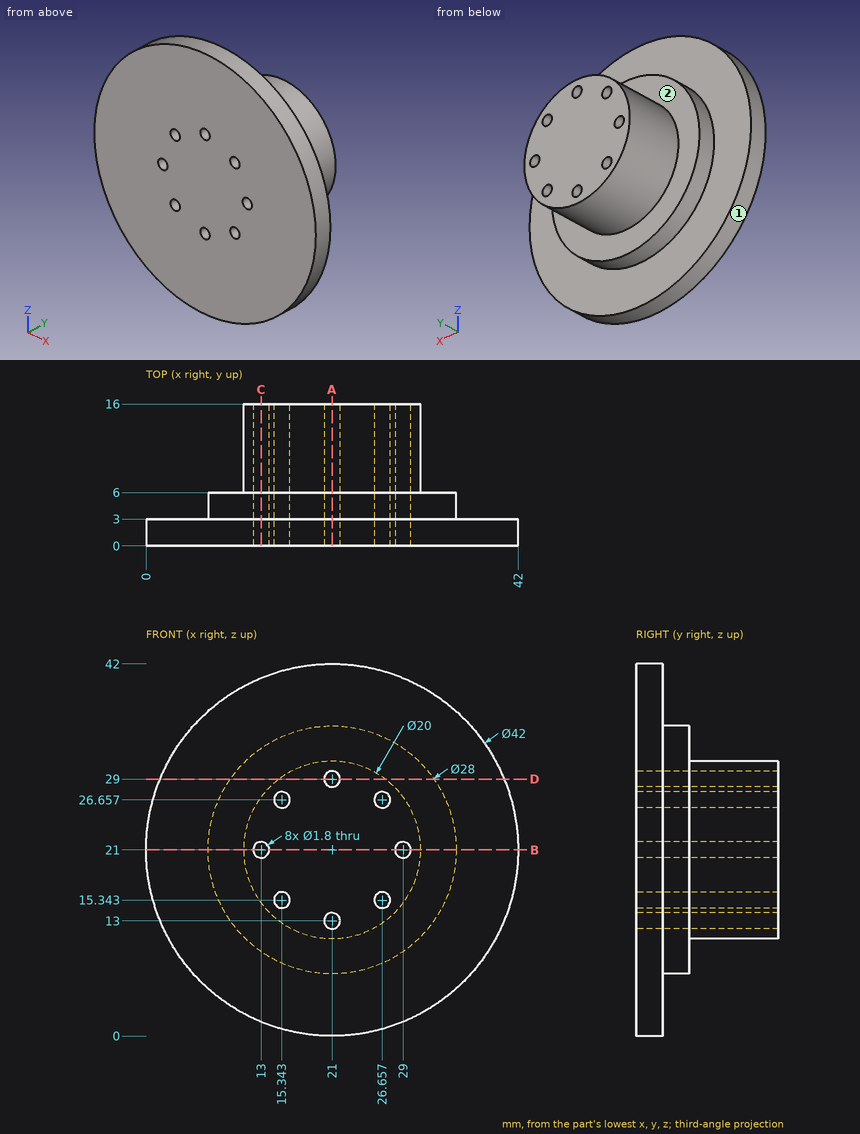
The drawing under review shows one solid part. Ordinate dimensions are in mm from its lowest x, y, z. A direction names the side the tool comes from. Coordinates: 2 decimals unless noted, no trailing zeros. Loops run counter-clockwise (first coordinate to the right, second up) from the corner with the lowest first, then second, coordinate; pieces in that order, holes last. Notation, with made-up numbers: (-24, 44.25) - (3, 44.25) arc R11 ccw to (3, 50.25) - close; hole circle Ø8 at (-39, 14.5). An arc over 180 degrees is marked (long way). Use CSV: the item, a comma, the result in double quotes. Start each with the question number.
1. Add section B-B on z = 21. Give the boundary of the cut face in (x, y).
2. Clearance check with flat-ended pins moving along their axes: pin 1 (2 mm diameter, centred on y = 12, z = 17.5, fed in from -X); pin 2 (4 mm diameter, centred on x = 25.5, z = 6.5, fed in from +Y); pin 3 (5 mm diameter, centred on y = 4, z = 14, fed in from -X). State where each tip first meets the part, or that it passes through.
3. Add section A-A on x = 21. Give the boundary of the cut face in (y, z).
4. Add section D-D on z = 29. Give the boundary of the cut face in (x, y).
5. To check wall thickness, follow probe 1 along Z at (x, y) = (21, 3.75); probe 2 along Y at (x, z) = (36.5, 32); probe 3 along X at (y, z) = (6.5, 16). State the ranges of each line that lie inside material, in increasing order.
6. Add section C-C on x = 13. Give the boundary of the cut face in (y, z), plus the area to 3 significant figures.
7. For the marked faces 1 and 2, list the 3-axis set-ups (+Z, -Z, +X, -X, +Y, -Y) from which the entire face can be reached by the end or side of a thin tool; tool diameter is ignored.
Resolved:
1,outline,"(0, 0) - (12.1, 0) - (12.1, 16) - (11, 16) - (11, 6) - (7, 6) - (7, 3) - (0, 3) - close; (13.9, 0) - (28.1, 0) - (28.1, 16) - (13.9, 16) - close; (29.9, 0) - (42, 0) - (42, 3) - (35, 3) - (35, 6) - (31, 6) - (31, 16) - (29.9, 16) - close"
2,pin 1,"x = 11.32"
2,pin 2,"y = 6"
2,pin 3,"x = 0.53"
3,outline,"(0, 0) - (3, 0) - (3, 7) - (6, 7) - (6, 11) - (16, 11) - (16, 12.1) - (0, 12.1) - close; (0, 13.9) - (16, 13.9) - (16, 28.1) - (0, 28.1) - close; (0, 29.9) - (16, 29.9) - (16, 31) - (6, 31) - (6, 35) - (3, 35) - (3, 42) - (0, 42) - close"
4,outline,"(1.58, 0) - (20.1, 0) - (20.1, 16) - (15, 16) - (15, 6) - (9.51, 6) - (9.51, 3) - (1.58, 3) - close; (21.9, 0) - (40.42, 0) - (40.42, 3) - (32.49, 3) - (32.49, 6) - (27, 6) - (27, 16) - (21.9, 16) - close"
5,probe 1,"7 to 12.1, 13.9 to 28.1, 29.9 to 35"
5,probe 2,"0 to 3"
5,probe 3,"12.34 to 14.73, 15.96 to 26.04, 27.27 to 29.66"
6,outline,"(0, 1.58) - (3, 1.58) - (3, 9.51) - (6, 9.51) - (6, 15) - (16, 15) - (16, 20.1) - (0, 20.1) - close; (0, 21.9) - (16, 21.9) - (16, 27) - (6, 27) - (6, 32.49) - (3, 32.49) - (3, 40.42) - (0, 40.42) - close"
6,area,"277 mm2"
7,face 1,"+Y, -Y"
7,face 2,"+Y"
